Design review of the part built by this model. Coordinates are the model's own, in mm. Face numbers are marked on the shaded views. A direction names the side the tool comes from. Give positions to 0.01 mm unless a question says otherwise; leave off trailing zeros. Loops run counter-clockwise (first coordinate to the right, second up) from the corner with the lowest first, then second, coordinate; pieces in that order, holes last. Notation, with made-up numbers: (41.25, -12.5) -> (61.25, -12.5) arc R22 ccw to (61.25, 10.5) -> close; hole circle Ø2 at (58, 83.25). An arc over 180 degrees is marked (long way). Answer in a Markdown table with one row per item. Add a question column.
(1) Consider section B-B on z = -4. Count the separate pieces of the cut face and the enclosed holes in it, then the cut area to 3 significant figures.
(2) Draft analysis for pull direction Y (two halves, no side actions). For the marked faces 4, 5 and 6, state which applies: +Y half, -Y half, draft (parallel to the pull), parting line (faces both ways), or undercut.
(3) For the marked faces 1, 2 and 3, list the 3-axis set-ups (+Z, -Z, +X, -X, +Y, -Y) from which the entire face can be reached by the end or side of a thin tool; tool diameter is ignored.
(4) Consider section A-A on y = -8.8. Write out the cut boundary in (x, z), then the cut area to 3 significant figures.
(5) Consider section C-C on y = -26.25. Write out the cut boundary in (x, z), then the cut area to 3 significant figures.
(6) For pin 1 (1.1 mm diameter, centred on x = 12.1, y = -29.4, fed in from +Z); pin 2 (1 mm diameter, centred on y = -5.95, z = -1.25, fed in from +X); pin 3 (2 mm diameter, centred on x = 2.5, z = 1, fed in from +Y); pin 4 (0.6 mm diameter, centred on x = -12, y = -4, fed in from -Z), all flat-tipped, find the tip position at first contact; note any pin that passes through.
(7) For line 1 (X direction, y = -50, z = -3.85); line 2 (Z direction, x = -11.1, y = -33.9); line 3 (X direction, y = -39.7, z = 4.1), list the stretches that pass through material, from the lowest coordinate up.
(8) Consider section D-D on x = -8.5. Write out the cut boundary in (y, z), then the cut area to 3 significant figures.
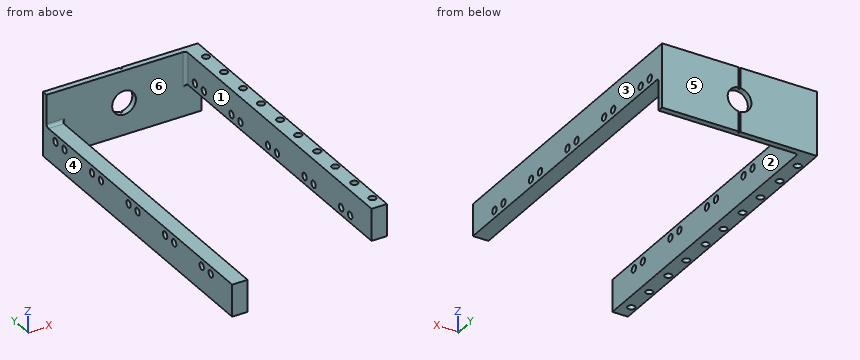
from build123d import *

# Parameters (mm, degrees)
SKETCH1_W              = 26.1
SKETCH1_H              = 10.8
EXTRUDE_284_DEPTH      = 1
SKETCH2_W              = 2.6
SKETCH2_H              = 5.4
EXTRUDE_422_DEPTH      = 51.5
SKETCH3_W              = 2.6
SKETCH3_H              = 5.4
EXTRUDE_634_DEPTH      = 51.5
SKETCH4_R              = 0.6
F_1_TIP_DEPTH          = 2
SKETCH5_R              = 0.6
F_2_TIP_DEPTH          = 2
SKETCH6_R              = 0.6
F_3_TIP_DEPTH          = 2
SKETCH7_R              = 0.6
F_4_TIP_DEPTH          = 2
SKETCH8_R              = 0.6
F_5_TIP_DEPTH          = 2
SKETCH9_R              = 0.6
F_6_TIP_DEPTH          = 2
SKETCH10_R             = 0.6
F_7_TIP_DEPTH          = 2
SKETCH11_R             = 0.6
F_8_TIP_DEPTH          = 2
SKETCH12_R             = 0.6
F_9_TIP_DEPTH          = 2
SKETCH13_R             = 0.6
F_10_TIP_DEPTH         = 2
SKETCH14_R             = 0.6
F_1_SAMPLE_DEPTH       = 2.6
SKETCH15_R             = 0.6
F_2_SAMPLE_DEPTH       = 2.6
SKETCH16_R             = 0.6
F_3_SAMPLE_DEPTH       = 2.6
SKETCH17_R             = 0.6
F_4_SAMPLE_DEPTH       = 2.6
SKETCH18_R             = 0.6
F_5_SAMPLE_DEPTH       = 2.6
SKETCH19_R             = 0.6
F_6_SAMPLE_DEPTH       = 2.6
SKETCH20_R             = 0.6
F_7_SAMPLE_DEPTH       = 2.6
SKETCH21_R             = 0.6
F_8_SAMPLE_DEPTH       = 2.6
SKETCH22_R             = 0.6
F_9_SAMPLE_DEPTH       = 2.6
SKETCH23_R             = 0.6
F_10_SAMPLE_DEPTH      = 2.6
SKETCH24_R             = 0.6
F_1_SAMPLE_2_DEPTH     = 2.6
SKETCH25_R             = 0.6
F_2_SAMPLE_2_DEPTH     = 2.6
SKETCH26_R             = 0.6
F_3_SAMPLE_2_DEPTH     = 2.6
SKETCH27_R             = 0.6
F_4_SAMPLE_2_DEPTH     = 2.6
SKETCH28_R             = 0.6
F_5_SAMPLE_2_DEPTH     = 2.6
SKETCH29_R             = 0.6
F_6_SAMPLE_2_DEPTH     = 2.6
SKETCH30_R             = 0.6
F_7_SAMPLE_2_DEPTH     = 2.6
SKETCH31_R             = 0.6
F_8_SAMPLE_2_DEPTH     = 2.6
SKETCH32_R             = 0.6
F_9_SAMPLE_2_DEPTH     = 2.6
SKETCH33_R             = 0.6
F_10_SAMPLE_2_DEPTH    = 2.6
SKETCH34_R             = 0.6
F_1_TIP_2_DEPTH        = 2
SKETCH35_R             = 0.6
F_2_TIP_2_DEPTH        = 2
SKETCH36_R             = 0.6
F_3_TIP_2_DEPTH        = 2
SKETCH37_R             = 0.6
F_4_TIP_2_DEPTH        = 2
SKETCH38_R             = 0.6
F_5_TIP_2_DEPTH        = 2
SKETCH39_R             = 0.6
F_6_TIP_2_DEPTH        = 2
SKETCH40_R             = 0.6
F_7_TIP_2_DEPTH        = 2
SKETCH41_R             = 0.6
F_8_TIP_2_DEPTH        = 2
SKETCH42_R             = 0.6
F_9_TIP_2_DEPTH        = 2
SKETCH43_R             = 0.6
F_10_TIP_2_DEPTH       = 2
SKETCH44_R             = 2
CUT_EXTRUDE_M4_DEPTH   = 3
FILLET1_R              = 0.5
FILLET2_R              = 0.5
SKETCH45_W             = 0.3
SKETCH45_H             = 10.8
CUT_EXTRUDE_9209_DEPTH = 0.3


with BuildPart() as part:
    # Sketch1 → Extrude 284 (new body)
    with BuildSketch(Plane(origin=(0, 0, 0), x_dir=(1, 0, 0), z_dir=(0, 1, 0))):
        Rectangle(SKETCH1_W, SKETCH1_H)
    extrude(amount=-EXTRUDE_284_DEPTH)

    # Sketch2 → Extrude 422 (add)
    with BuildSketch(Plane.XZ.offset(1)):
        with Locations((11.75, 2.7)):
            Rectangle(SKETCH2_W, SKETCH2_H)
    extrude(amount=EXTRUDE_422_DEPTH)

    # Sketch3 → Extrude 634 (add)
    with BuildSketch(Plane.XZ.offset(1)):
        with Locations((-11.75, -2.7)):
            Rectangle(SKETCH3_W, SKETCH3_H)
    extrude(amount=EXTRUDE_634_DEPTH)

    # Sketch4 → 1-tip (cut)
    with BuildSketch(Plane.XY.offset(5.4)):
        with Locations((12.1, -3.8)):
            Circle(SKETCH4_R)
    extrude(amount=-F_1_TIP_DEPTH, mode=Mode.SUBTRACT)

    # Sketch5 → 2-tip (cut)
    with BuildSketch(Plane.XY.offset(5.4)):
        with Locations((12.1, -8.8)):
            Circle(SKETCH5_R)
    extrude(amount=-F_2_TIP_DEPTH, mode=Mode.SUBTRACT)

    # Sketch6 → 3-tip (cut)
    with BuildSketch(Plane.XY.offset(5.4)):
        with Locations((12.1, -14.1)):
            Circle(SKETCH6_R)
    extrude(amount=-F_3_TIP_DEPTH, mode=Mode.SUBTRACT)

    # Sketch7 → 4-tip (cut)
    with BuildSketch(Plane.XY.offset(5.4)):
        with Locations((12.1, -19.1)):
            Circle(SKETCH7_R)
    extrude(amount=-F_4_TIP_DEPTH, mode=Mode.SUBTRACT)

    # Sketch8 → 5-tip (cut)
    with BuildSketch(Plane.XY.offset(5.4)):
        with Locations((12.1, -24.4)):
            Circle(SKETCH8_R)
    extrude(amount=-F_5_TIP_DEPTH, mode=Mode.SUBTRACT)

    # Sketch9 → 6-tip (cut)
    with BuildSketch(Plane.XY.offset(5.4)):
        with Locations((12.1, -29.4)):
            Circle(SKETCH9_R)
    extrude(amount=-F_6_TIP_DEPTH, mode=Mode.SUBTRACT)

    # Sketch10 → 7-tip (cut)
    with BuildSketch(Plane.XY.offset(5.4)):
        with Locations((12.1, -34.7)):
            Circle(SKETCH10_R)
    extrude(amount=-F_7_TIP_DEPTH, mode=Mode.SUBTRACT)

    # Sketch11 → 8-tip (cut)
    with BuildSketch(Plane.XY.offset(5.4)):
        with Locations((12.1, -39.7)):
            Circle(SKETCH11_R)
    extrude(amount=-F_8_TIP_DEPTH, mode=Mode.SUBTRACT)

    # Sketch12 → 9-tip (cut)
    with BuildSketch(Plane.XY.offset(5.4)):
        with Locations((12.1, -45)):
            Circle(SKETCH12_R)
    extrude(amount=-F_9_TIP_DEPTH, mode=Mode.SUBTRACT)

    # Sketch13 → 10-tip (cut)
    with BuildSketch(Plane.XY.offset(5.4)):
        with Locations((12.1, -50)):
            Circle(SKETCH13_R)
    extrude(amount=-F_10_TIP_DEPTH, mode=Mode.SUBTRACT)

    # Sketch14 → 1-sample (cut)
    with BuildSketch(Plane.ZY.offset(-10.45)):
        with Locations((1.25, -3.45)):
            Circle(SKETCH14_R)
    extrude(amount=-F_1_SAMPLE_DEPTH, mode=Mode.SUBTRACT)

    # Sketch15 → 2-sample (cut)
    with BuildSketch(Plane.ZY.offset(-10.45)):
        with Locations((1.25, -5.95)):
            Circle(SKETCH15_R)
    extrude(amount=-F_2_SAMPLE_DEPTH, mode=Mode.SUBTRACT)

    # Sketch16 → 3-sample (cut)
    with BuildSketch(Plane.ZY.offset(-10.45)):
        with Locations((1.25, -13.6)):
            Circle(SKETCH16_R)
    extrude(amount=-F_3_SAMPLE_DEPTH, mode=Mode.SUBTRACT)

    # Sketch17 → 4-sample (cut)
    with BuildSketch(Plane.ZY.offset(-10.45)):
        with Locations((1.25, -16.1)):
            Circle(SKETCH17_R)
    extrude(amount=-F_4_SAMPLE_DEPTH, mode=Mode.SUBTRACT)

    # Sketch18 → 5-sample (cut)
    with BuildSketch(Plane.ZY.offset(-10.45)):
        with Locations((1.25, -23.75)):
            Circle(SKETCH18_R)
    extrude(amount=-F_5_SAMPLE_DEPTH, mode=Mode.SUBTRACT)

    # Sketch19 → 6-sample (cut)
    with BuildSketch(Plane.ZY.offset(-10.45)):
        with Locations((1.25, -26.25)):
            Circle(SKETCH19_R)
    extrude(amount=-F_6_SAMPLE_DEPTH, mode=Mode.SUBTRACT)

    # Sketch20 → 7-sample (cut)
    with BuildSketch(Plane.ZY.offset(-10.45)):
        with Locations((1.25, -33.9)):
            Circle(SKETCH20_R)
    extrude(amount=-F_7_SAMPLE_DEPTH, mode=Mode.SUBTRACT)

    # Sketch21 → 8-sample (cut)
    with BuildSketch(Plane.ZY.offset(-10.45)):
        with Locations((1.25, -36.4)):
            Circle(SKETCH21_R)
    extrude(amount=-F_8_SAMPLE_DEPTH, mode=Mode.SUBTRACT)

    # Sketch22 → 9-sample (cut)
    with BuildSketch(Plane.ZY.offset(-10.45)):
        with Locations((1.25, -44.05)):
            Circle(SKETCH22_R)
    extrude(amount=-F_9_SAMPLE_DEPTH, mode=Mode.SUBTRACT)

    # Sketch23 → 10-sample (cut)
    with BuildSketch(Plane.ZY.offset(-10.45)):
        with Locations((1.25, -46.55)):
            Circle(SKETCH23_R)
    extrude(amount=-F_10_SAMPLE_DEPTH, mode=Mode.SUBTRACT)

    # Sketch24 → 1-sample 2 (cut)
    with BuildSketch(Plane(origin=(-10.45, 0, 0), x_dir=(0, 0, -1), z_dir=(1, 0, 0))):
        with Locations((1.25, -3.45)):
            Circle(SKETCH24_R)
    extrude(amount=-F_1_SAMPLE_2_DEPTH, mode=Mode.SUBTRACT)

    # Sketch25 → 2-sample 2 (cut)
    with BuildSketch(Plane(origin=(-10.45, 0, 0), x_dir=(0, 0, -1), z_dir=(1, 0, 0))):
        with Locations((1.25, -5.95)):
            Circle(SKETCH25_R)
    extrude(amount=-F_2_SAMPLE_2_DEPTH, mode=Mode.SUBTRACT)

    # Sketch26 → 3-sample 2 (cut)
    with BuildSketch(Plane(origin=(-10.45, 0, 0), x_dir=(0, 0, -1), z_dir=(1, 0, 0))):
        with Locations((1.25, -13.6)):
            Circle(SKETCH26_R)
    extrude(amount=-F_3_SAMPLE_2_DEPTH, mode=Mode.SUBTRACT)

    # Sketch27 → 4-sample 2 (cut)
    with BuildSketch(Plane(origin=(-10.45, 0, 0), x_dir=(0, 0, -1), z_dir=(1, 0, 0))):
        with Locations((1.25, -16.1)):
            Circle(SKETCH27_R)
    extrude(amount=-F_4_SAMPLE_2_DEPTH, mode=Mode.SUBTRACT)

    # Sketch28 → 5-sample 2 (cut)
    with BuildSketch(Plane(origin=(-10.45, 0, 0), x_dir=(0, 0, -1), z_dir=(1, 0, 0))):
        with Locations((1.25, -23.75)):
            Circle(SKETCH28_R)
    extrude(amount=-F_5_SAMPLE_2_DEPTH, mode=Mode.SUBTRACT)

    # Sketch29 → 6-sample 2 (cut)
    with BuildSketch(Plane(origin=(-10.45, 0, 0), x_dir=(0, 0, -1), z_dir=(1, 0, 0))):
        with Locations((1.25, -26.25)):
            Circle(SKETCH29_R)
    extrude(amount=-F_6_SAMPLE_2_DEPTH, mode=Mode.SUBTRACT)

    # Sketch30 → 7-sample 2 (cut)
    with BuildSketch(Plane(origin=(-10.45, 0, 0), x_dir=(0, 0, -1), z_dir=(1, 0, 0))):
        with Locations((1.25, -33.9)):
            Circle(SKETCH30_R)
    extrude(amount=-F_7_SAMPLE_2_DEPTH, mode=Mode.SUBTRACT)

    # Sketch31 → 8-sample 2 (cut)
    with BuildSketch(Plane(origin=(-10.45, 0, 0), x_dir=(0, 0, -1), z_dir=(1, 0, 0))):
        with Locations((1.25, -36.4)):
            Circle(SKETCH31_R)
    extrude(amount=-F_8_SAMPLE_2_DEPTH, mode=Mode.SUBTRACT)

    # Sketch32 → 9-sample 2 (cut)
    with BuildSketch(Plane(origin=(-10.45, 0, 0), x_dir=(0, 0, -1), z_dir=(1, 0, 0))):
        with Locations((1.25, -44.05)):
            Circle(SKETCH32_R)
    extrude(amount=-F_9_SAMPLE_2_DEPTH, mode=Mode.SUBTRACT)

    # Sketch33 → 10-sample 2 (cut)
    with BuildSketch(Plane(origin=(-10.45, 0, 0), x_dir=(0, 0, -1), z_dir=(1, 0, 0))):
        with Locations((1.25, -46.55)):
            Circle(SKETCH33_R)
    extrude(amount=-F_10_SAMPLE_2_DEPTH, mode=Mode.SUBTRACT)

    # Sketch34 → 1-tip 2 (cut)
    with BuildSketch(Plane(origin=(0, 0, -5.4), x_dir=(-1, 0, 0), z_dir=(0, 0, -1))):
        with Locations((12.1, -3.8)):
            Circle(SKETCH34_R)
    extrude(amount=-F_1_TIP_2_DEPTH, mode=Mode.SUBTRACT)

    # Sketch35 → 2-tip 2 (cut)
    with BuildSketch(Plane(origin=(0, 0, -5.4), x_dir=(-1, 0, 0), z_dir=(0, 0, -1))):
        with Locations((12.1, -8.8)):
            Circle(SKETCH35_R)
    extrude(amount=-F_2_TIP_2_DEPTH, mode=Mode.SUBTRACT)

    # Sketch36 → 3-tip 2 (cut)
    with BuildSketch(Plane(origin=(0, 0, -5.4), x_dir=(-1, 0, 0), z_dir=(0, 0, -1))):
        with Locations((12.1, -14.1)):
            Circle(SKETCH36_R)
    extrude(amount=-F_3_TIP_2_DEPTH, mode=Mode.SUBTRACT)

    # Sketch37 → 4-tip 2 (cut)
    with BuildSketch(Plane(origin=(0, 0, -5.4), x_dir=(-1, 0, 0), z_dir=(0, 0, -1))):
        with Locations((12.1, -19.1)):
            Circle(SKETCH37_R)
    extrude(amount=-F_4_TIP_2_DEPTH, mode=Mode.SUBTRACT)

    # Sketch38 → 5-tip 2 (cut)
    with BuildSketch(Plane(origin=(0, 0, -5.4), x_dir=(-1, 0, 0), z_dir=(0, 0, -1))):
        with Locations((12.1, -24.4)):
            Circle(SKETCH38_R)
    extrude(amount=-F_5_TIP_2_DEPTH, mode=Mode.SUBTRACT)

    # Sketch39 → 6-tip 2 (cut)
    with BuildSketch(Plane(origin=(0, 0, -5.4), x_dir=(-1, 0, 0), z_dir=(0, 0, -1))):
        with Locations((12.1, -29.4)):
            Circle(SKETCH39_R)
    extrude(amount=-F_6_TIP_2_DEPTH, mode=Mode.SUBTRACT)

    # Sketch40 → 7-tip 2 (cut)
    with BuildSketch(Plane(origin=(0, 0, -5.4), x_dir=(-1, 0, 0), z_dir=(0, 0, -1))):
        with Locations((12.1, -34.7)):
            Circle(SKETCH40_R)
    extrude(amount=-F_7_TIP_2_DEPTH, mode=Mode.SUBTRACT)

    # Sketch41 → 8-tip 2 (cut)
    with BuildSketch(Plane(origin=(0, 0, -5.4), x_dir=(-1, 0, 0), z_dir=(0, 0, -1))):
        with Locations((12.1, -39.7)):
            Circle(SKETCH41_R)
    extrude(amount=-F_8_TIP_2_DEPTH, mode=Mode.SUBTRACT)

    # Sketch42 → 9-tip 2 (cut)
    with BuildSketch(Plane(origin=(0, 0, -5.4), x_dir=(-1, 0, 0), z_dir=(0, 0, -1))):
        with Locations((12.1, -45)):
            Circle(SKETCH42_R)
    extrude(amount=-F_9_TIP_2_DEPTH, mode=Mode.SUBTRACT)

    # Sketch43 → 10-tip 2 (cut)
    with BuildSketch(Plane(origin=(0, 0, -5.4), x_dir=(-1, 0, 0), z_dir=(0, 0, -1))):
        with Locations((12.1, -50)):
            Circle(SKETCH43_R)
    extrude(amount=-F_10_TIP_2_DEPTH, mode=Mode.SUBTRACT)

    # Sketch44 → Cut-Extrude M4 (cut)
    with BuildSketch(Plane(origin=(0, 0, 0), x_dir=(1, 0, 0), z_dir=(0, 1, 0))):
        with Locations(Location((0, 0, 0), (0, 0, 270))):
            Circle(SKETCH44_R)
    extrude(amount=-CUT_EXTRUDE_M4_DEPTH, mode=Mode.SUBTRACT)

    # Fillet1
    fillet1_edges = [part.edges().sort_by_distance(p)[0] for p in [
        (10.45, -1, 2.7),
        (-10.45, -1, -2.7),
    ]]
    fillet(fillet1_edges, radius=FILLET1_R)

    # Fillet2
    fillet2_edges = [part.edges().sort_by_distance(p)[0] for p in [
        (11.5, -1, 0),
        (-11.5, -1, 0),
    ]]
    fillet(fillet2_edges, radius=FILLET2_R)

    # Sketch45 → Cut-Extrude 9209 (cut)
    with BuildSketch(Plane(origin=(0, 0, 0), x_dir=(1, 0, 0), z_dir=(0, 1, 0))):
        Rectangle(SKETCH45_W, SKETCH45_H)
    extrude(amount=-CUT_EXTRUDE_9209_DEPTH, mode=Mode.SUBTRACT)


solid = part.part
Values follow:
| question | item | result |
|---|---|---|
| 1 | separate pieces | 1 |
| 1 | enclosed holes | 10 |
| 1 | area | 149 mm2 |
| 2 | face 4 | draft |
| 2 | face 5 | +Y half |
| 2 | face 6 | -Y half |
| 3 | face 1 | +Z, -Z, -X, -Y |
| 3 | face 2 | +Z, -Z, +X, -Y |
| 3 | face 3 | +Z, -Z, +X, +Y, -Y |
| 4 | outline | (-13.05, -5.4) -> (-12.7, -5.4) -> (-12.7, -3.4) -> (-11.5, -3.4) -> (-11.5, -5.4) -> (-10.45, -5.4) -> (-10.45, 0) -> (-13.05, 0) -> close; (10.45, 0) -> (13.05, 0) -> (13.05, 5.4) -> (12.7, 5.4) -> (12.7, 3.4) -> (11.5, 3.4) -> (11.5, 5.4) -> (10.45, 5.4) -> close |
| 4 | area | 23.3 mm2 |
| 5 | outline | (-13.05, -5.4) -> (-10.45, -5.4) -> (-10.45, -1.85) -> (-13.05, -1.85) -> close; (-13.05, -0.65) -> (-10.45, -0.65) -> (-10.45, 0) -> (-13.05, 0) -> close; (10.45, 0) -> (13.05, 0) -> (13.05, 0.65) -> (10.45, 0.65) -> close; (10.45, 1.85) -> (13.05, 1.85) -> (13.05, 5.4) -> (10.45, 5.4) -> close |
| 5 | area | 21.8 mm2 |
| 6 | pin 1 | z = 3.4 |
| 6 | pin 2 | through |
| 6 | pin 3 | y = 0 |
| 6 | pin 4 | z = -3.4 |
| 7 | line 1 | -13.05 to -12.7, -11.5 to -10.45 |
| 7 | line 2 | -5.4 to -1.85, -0.65 to 0 |
| 7 | line 3 | 10.45 to 11.5, 12.7 to 13.05 |
| 8 | outline | (-1, -5.4) -> (0, -5.4) -> (0, 5.4) -> (-1, 5.4) -> close |
| 8 | area | 10.8 mm2 |
